CAD build for the part. Positions are in the model's coordinates, mm. A direction names the side the tool comes from. Coordinates: 2 decimals unless noted, no trailing zeros. Order: outer loops, then holes, each group sorted by start corner. A loop starts at its lowest first (then second) coordinate and runs counter-clockwise, first axis right, second up. Notation, with made-up numbers: (34, 36.5) - (88, 36.5) arc R29 ccw to (88, 67.5) - close; hole circle Ø6 at (59.25, 48). An arc over 180 degrees is marked (long way). Write each question's results on one line, items separated by ' | '. Start each with the question number.
Q1. Which spindle directions (+Z, -Z, +X, -X, +Y, -Y) get a long thin tool onto all of the face, cutting with end or side? Do faces 1 (the flat face through (-1.27, 6, 0)), 2 (the flat face through (0, 6.452, 19)), 3 (the flat face through (0, 5.588, 22)). Say none if no direction does.
Q2. Wall check: probe 1 along X at (y, z) = (6.25, -17); probe 2 along Y at (x, z) = (-1, 14.5); probe 3 along X at (y, z) = (7.75, 0). Give the ranges that are in metal, low to high.
Q3. Band-saw the part on B-B, the plane x = 0.5. Write the cut outline in (y, z) (3 decimals).
Q4. Pull direction X, two halves, no side cores. Call faces 4 (the flat face through (-16.833, 7.599, 0.32)), 5 (the flat face through (17.297, 3, 0)), 6 (the flat face through (0, 3, -22.86)), 7 (the flat face through (0, 5.588, -22)): released by +X, released by -X, zero draft, split by the parting line, or undercut.
Q5. Pin check, flat tips, straight feed: P1, Ø1.3, axis at x = 0.5, z = -22.5, coming from the +Y side; P2, Ø1.3, axis at x = 0, z = 19.5, coming from the +Y side. Stop position of each tip, or through.
Q6. Band-saw the part on A-A, the plane z = -13.5. Write the cut outline in (x, y).
```python
from build123d import *

# Parameters (mm, degrees)
BOSS_EXTRUDE1_DEPTH   = 22.86
CHAMFER1_SIZE         = 1.5875
CHAMFER1_SIZE2        = 0.916543552
CHAMFER1_PART_2_SIZE  = 1.5875
CHAMFER1_PART_2_SIZE2 = 0.916543552
CHAMFER1_PART_3_SIZE  = 1.5875
CHAMFER1_PART_3_SIZE2 = 0.916543552
CHAMFER1_PART_4_SIZE  = 1.5875
CHAMFER1_PART_4_SIZE2 = 0.916543552
CHAMFER1_PART_5_SIZE  = 1.5875
CHAMFER1_PART_5_SIZE2 = 0.916543552
CHAMFER1_PART_6_SIZE  = 1.5875
CHAMFER1_PART_6_SIZE2 = 0.916543552
BOSS_EXTRUDE2_START   = 17.145
SKETCH2_W             = 2.54
SKETCH2_H             = 0.8636
BOSS_EXTRUDE2_DEPTH   = 4.064


with BuildPart() as part:
    # Sketch1 → Boss-Extrude1 (new body, symmetric)
    with BuildSketch(Plane.XY):
        Polygon((-17.2974, 0), (17.2974, 0), (17.2974, 8.382), (1.27, 8.382), (1.27, 5.588), (-1.27, 5.588), (-1.27, 8.382), (-17.2974, 8.382), align=None)
    extrude(amount=BOSS_EXTRUDE1_DEPTH, both=True)

    # Chamfer1
    chamfer1_edges = [part.edges().sort_by_distance(p)[0] for p in [
        (9.2837, 8.382, -22.86),
        (-9.2837, 8.382, -22.86),
    ]]
    chamfer1_side = [part.faces().sort_by_distance(p)[0] for p in [
        (0, 4.120904666, -22.86),
    ]]
    chamfer(chamfer1_edges, length=CHAMFER1_SIZE, length2=CHAMFER1_SIZE2, reference=chamfer1_side[0])

    # Chamfer1 part 2
    chamfer1_part_2_edges = [part.edges().sort_by_distance(p)[0] for p in [
        (17.2974, 8.382, 0),
    ]]
    chamfer1_part_2_side = [part.faces().sort_by_distance(p)[0] for p in [
        (17.2974, 4.191, 0),
    ]]
    chamfer(chamfer1_part_2_edges, length=CHAMFER1_PART_2_SIZE, length2=CHAMFER1_PART_2_SIZE2, reference=chamfer1_part_2_side[0])

    # Chamfer1 part 3
    chamfer1_part_3_edges = [part.edges().sort_by_distance(p)[0] for p in [
        (-17.2974, 8.382, 0),
    ]]
    chamfer1_part_3_side = [part.faces().sort_by_distance(p)[0] for p in [
        (-17.2974, 4.191, 0),
    ]]
    chamfer(chamfer1_part_3_edges, length=CHAMFER1_PART_3_SIZE, length2=CHAMFER1_PART_3_SIZE2, reference=chamfer1_part_3_side[0])

    # Chamfer1 part 4
    chamfer1_part_4_edges = [part.edges().sort_by_distance(p)[0] for p in [
        (-1.27, 8.382, 0),
    ]]
    chamfer1_part_4_side = [part.faces().sort_by_distance(p)[0] for p in [
        (-1.27, 6.985, 0),
    ]]
    chamfer(chamfer1_part_4_edges, length=CHAMFER1_PART_4_SIZE, length2=CHAMFER1_PART_4_SIZE2, reference=chamfer1_part_4_side[0])

    # Chamfer1 part 5
    chamfer1_part_5_edges = [part.edges().sort_by_distance(p)[0] for p in [
        (1.27, 8.382, 0),
    ]]
    chamfer1_part_5_side = [part.faces().sort_by_distance(p)[0] for p in [
        (1.27, 6.985, 0),
    ]]
    chamfer(chamfer1_part_5_edges, length=CHAMFER1_PART_5_SIZE, length2=CHAMFER1_PART_5_SIZE2, reference=chamfer1_part_5_side[0])

    # Chamfer1 part 6
    chamfer1_part_6_edges = [part.edges().sort_by_distance(p)[0] for p in [
        (-9.2837, 8.382, 22.86),
        (9.2837, 8.382, 22.86),
    ]]
    chamfer1_part_6_side = [part.faces().sort_by_distance(p)[0] for p in [
        (0, 4.120904666, 22.86),
    ]]
    chamfer(chamfer1_part_6_edges, length=CHAMFER1_PART_6_SIZE, length2=CHAMFER1_PART_6_SIZE2, reference=chamfer1_part_6_side[0])

    # Sketch2 → Boss-Extrude2 (add)
    with BuildSketch(Plane.XY.offset(BOSS_EXTRUDE2_START)):
        with Locations((0, 6.0198)):
            Rectangle(SKETCH2_W, SKETCH2_H)
    boss_extrude2 = extrude(amount=BOSS_EXTRUDE2_DEPTH)

    # Mirror1: Boss-Extrude2 across plane
    add(boss_extrude2.mirror(Plane.XY))


solid = part.part
```
Results below:
1) face 1: +Y | face 2: +Z, -Z, +Y | face 3: +Z, +Y
2) probe 1: x = -17.3 to -1.27, 1.27 to 17.3 | probe 2: y = 0 to 5.59 | probe 3: x = -16.75 to -1.82, 1.82 to 16.75
3) outline: (0, -22.86) - (5.588, -22.86) - (5.588, -21.209) - (6.452, -21.209) - (6.452, -17.145) - (5.588, -17.145) - (5.588, 17.145) - (6.452, 17.145) - (6.452, 21.209) - (5.588, 21.209) - (5.588, 22.86) - (0, 22.86) - close
4) face 4: released by -X | face 5: released by +X | face 6: zero draft | face 7: undercut
5) P1: stops at y = 5.59 | P2: stops at y = 6.45
6) outline: (-17.3, 0) - (17.3, 0) - (17.3, 6.79) - (16.38, 8.38) - (2.19, 8.38) - (1.27, 6.79) - (1.27, 5.59) - (-1.27, 5.59) - (-1.27, 6.79) - (-2.19, 8.38) - (-16.38, 8.38) - (-17.3, 6.79) - close
